Part model, mm, in its own coordinate system. Face numbers are marked on the shaded views. A direction names the side the tool comes from. Coordinates: 2 decimals unless noted, no trailing zeros. Loops run counter-clockwise (first coordinate to the right, second up) from the corner with the lowest first, then second, coordinate; pieces in that order, holes last. Notation, with made-up numbers: (-19, 71) -> (31, 71) arc R36 ccw to (31, 105) -> close; hole circle Ø8 at (61, 4). An arc over 180 degrees is marked (long way). One line per question, with ' | ' between items. Start each with the question number.
1) 3-axis set-ups, long thin cutter, end or side, ignore diameter. For the marked faces 1, 2, 3, 4 and 5: which of +Z, -Z, +X, -X, +Y, -Y reach the whole face in a straight line?
2) Cut at B-B (y = -2). List the corners of the cut face in (x, z), plus the area to 3 significant figures.
3) Probe L1, parallel to Z at x = -12.5, y = -29.8; L2, parallel to Y at x = 8, z = 50.95; L3, parallel to X at y = -30, z = 16. List the from-to ranges inside material, lowest first. Write a range as from..to.
4) Cut at D-D (x = 0). List the corners of the cut face in (y, z).
5) Drop flat-ended pins along their axis: pin 1 (6 mm diameter, centred on x = -10.5, z = 5, fed in from +Y); pin 2 (8 mm diameter, centred on x = -13.5, y = -12.5, fed in from +Z); pin 3 (5.5 mm diameter, centred on y = 1, z = 52.5, fed in from +X); pin 4 (2.5 mm diameter, centred on x = -8, y = 8, fed in from +Z). Give the stop position or say it passes through.
6) Two-plate mould, pull along Z, no slides. Class the marked faces 6, 7 and 8: released by +Z, released by -Z, zero draft, split by the parting line, or undercut.
7) Cut at A-A (x = 8). List the corners of the cut face in (y, z).
8) Cut at C-C (z = 0). List the corners of the cut face in (x, y), plus the area to 3 significant figures.
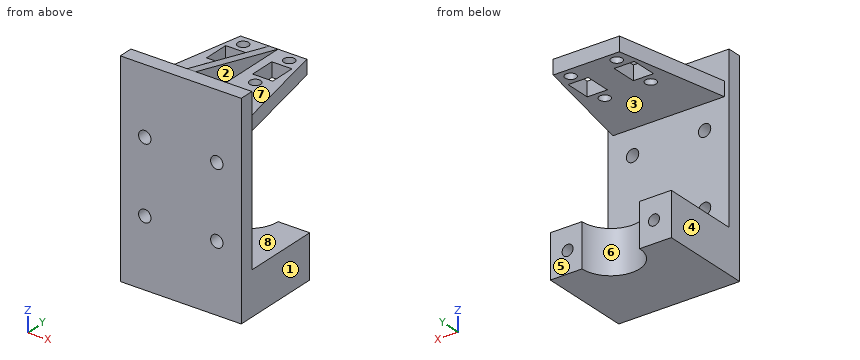
from build123d import *

# Parameters (mm, degrees)
MOTOR_MOUNT_SOLID_DEPTH              = 7.5
ENCODER_DISTANCE_SKETCH_W            = 50
ENCODER_DISTANCE_SKETCH_H            = 57
ENCODER_DISTANCE_SOLID_DEPTH         = 5
ENCODER_MOUNT_SKETCH_R               = 1.9
ENCODER_MOUNT_SKETCH_W               = 7
ENCODER_MOUNT_SKETCH_H               = 9
ENCODER_MOUNT_SOLID_DEPTH            = 5
MOTOR_CLAMP_MOUNTING_HOLES_SKETCH_R  = 1.9
MOTOR_CLAMP_MOUNTING_HOLES_CUT_DEPTH = 16
GUSSET_PLATE_SKETCH_W                = 50
GUSSET_PLATE_SKETCH_H                = 5
GUSSET_PLATE_SOLID_DEPTH             = 16.5
GUSSET_SOLID_DEPTH                   = 1.5
MOUNTING_PLATE_SKETCH_W              = 50
MOUNTING_PLATE_SKETCH_H              = 92
MOUNTING_PLATE_SKETCH_R              = 2.65
MOUNTING_PLATE_SOLID_DEPTH           = 5
MOUNTING_HOLES_CUT_DEPTH             = 101.440280764
MOUNTING_HOLES_CUT_DEPTH_BACK        = 101.440280764
MOUNTING_HOLE_SKETCH_R               = 2.65
MOUNTING_PLATE_TRIM_SKETCH_W         = 50
MOUNTING_PLATE_TRIM_SKETCH_H         = 13.5
MOUNTING_PLATE_TRIM_SKETCH_H_2       = 42
MOUNTING_PLATE_TRIM_SKETCH_W_2       = 23.5
MOUNTING_PLATE_TRIM_SKETCH_H_3       = 16.5
MOUNTING_PLATE_TRIM_CUT_DEPTH        = 2
CUT_EXTRUDE1_DEPTH                   = 102.917859083
CUT_EXTRUDE1_DEPTH_BACK              = 102.917859083
SKETCH2_W                            = 50
SKETCH2_H                            = 120
SKETCH2_W_2                          = 42
SKETCH2_H_2                          = 54.272597004
SKETCH3_W                            = 42
SKETCH3_H                            = 71.586450004
BOSS_EXTRUDE1_DEPTH                  = 5
CUT_EXTRUDE2_DEPTH                   = 78.722819275
CUT_EXTRUDE2_DEPTH_BACK              = 78.722819275
SKETCH4_R                            = 2.15


with BuildPart() as part:
    # Mouting Mount Sketch → Motor Mount Solid (new, symmetric)
    with BuildSketch(Plane.XY):
        with BuildLine():
            Line((-25, -55), (25, -55))
            Line((25, -55), (25, 0))
            Line((25, 0), (10, 0))
            ThreePointArc((10, 0), (0, -10), (-10, 0))
            Line((-10, 0), (-25, 0))
            Line((-25, 0), (-25, -55))
        make_face()
    extrude(amount=MOTOR_MOUNT_SOLID_DEPTH, both=True)

    # Encoder Distance Sketch → Encoder Distance Solid (add)
    with BuildSketch(Plane.XZ.offset(55)):
        with Locations((0, 21)):
            Rectangle(ENCODER_DISTANCE_SKETCH_W, ENCODER_DISTANCE_SKETCH_H)
    extrude(amount=ENCODER_DISTANCE_SOLID_DEPTH)

    # Encoder Mount Sketch → Encoder Mount Solid (add)
    with BuildSketch(Plane.XY.offset(49.5)):
        Polygon((-25, -60), (-25, -55), (-11.5, 11.5), (11.5, 11.5), (25, -55), (25, -60), align=None)
        with Locations((-8, 8)):
            Circle(ENCODER_MOUNT_SKETCH_R, mode=Mode.SUBTRACT)
        with Locations((8, 8)):
            Circle(ENCODER_MOUNT_SKETCH_R, mode=Mode.SUBTRACT)
        with Locations((-8, -8)):
            Circle(ENCODER_MOUNT_SKETCH_R, mode=Mode.SUBTRACT)
        with Locations((8, -8)):
            Circle(ENCODER_MOUNT_SKETCH_R, mode=Mode.SUBTRACT)
        with Locations((-8, 0)):
            Rectangle(ENCODER_MOUNT_SKETCH_W, ENCODER_MOUNT_SKETCH_H, mode=Mode.SUBTRACT)
        with Locations((8, 0)):
            Rectangle(ENCODER_MOUNT_SKETCH_W, ENCODER_MOUNT_SKETCH_H, mode=Mode.SUBTRACT)
    extrude(amount=ENCODER_MOUNT_SOLID_DEPTH)

    # Motor Clamp Mounting Holes Sketch → Motor Clamp Mounting Holes Cut (cut)
    with BuildSketch(Plane(origin=(0, 0, 0), x_dir=(1, 0, 0), z_dir=(0, 1, 0))):
        with Locations(Location((-15, 0, 0), (0, 0, 180))):
            Circle(MOTOR_CLAMP_MOUNTING_HOLES_SKETCH_R)
        with Locations(Location((15, 0, 0), (0, 0, 180))):
            Circle(MOTOR_CLAMP_MOUNTING_HOLES_SKETCH_R)
    extrude(amount=-MOTOR_CLAMP_MOUNTING_HOLES_CUT_DEPTH, mode=Mode.SUBTRACT)

    # Gusset Plate Sketch → Gusset Plate Solid (add)
    with BuildSketch(Plane.XY.offset(54.5)):
        with Locations((0, -57.5)):
            Rectangle(GUSSET_PLATE_SKETCH_W, GUSSET_PLATE_SKETCH_H)
    extrude(amount=GUSSET_PLATE_SOLID_DEPTH)

    # Gusset Sketch → Gusset Solid (add, symmetric)
    with BuildSketch(Plane(origin=(0, 0, 0), x_dir=(0, 0, -1), z_dir=(1, 0, 0))):
        Polygon((-54.5, 11.5), (-71, -55), (-54.5, -55), align=None)
    extrude(amount=GUSSET_SOLID_DEPTH, both=True)

    # Mounting Plate Sketch → Mounting Plate Solid (add)
    with BuildSketch(Plane(origin=(0, -55, 0), x_dir=(1, 0, 0), z_dir=(0, 1, 0))):
        with Locations((0, -25)):
            Rectangle(MOUNTING_PLATE_SKETCH_W, MOUNTING_PLATE_SKETCH_H)
        with Locations((-19, -65)):
            Circle(MOUNTING_PLATE_SKETCH_R, mode=Mode.SUBTRACT)
        with Locations((19, -65)):
            Circle(MOUNTING_PLATE_SKETCH_R, mode=Mode.SUBTRACT)
        with Locations(Location((-19, 15, 0), (0, 0, 270))):
            Circle(MOUNTING_PLATE_SKETCH_R, mode=Mode.SUBTRACT)
        with Locations(Location((19, 15, 0), (0, 0, 270))):
            Circle(MOUNTING_PLATE_SKETCH_R, mode=Mode.SUBTRACT)
    extrude(amount=-MOUNTING_PLATE_SOLID_DEPTH)

    # Mounting Hole Sketch → Mounting Holes Cut (cut, two sides: drawn at the far end of the back side and taken through both)
    with BuildSketch(Plane(origin=(0, -55, 0), x_dir=(1, 0, 0), z_dir=(0, 1, 0)).offset(-MOUNTING_HOLES_CUT_DEPTH_BACK)):
        with Locations(Location((-19, 15, 0), (0, 0, 270))):
            Circle(MOUNTING_HOLE_SKETCH_R)
        with Locations(Location((19, 15, 0), (0, 0, 270))):
            Circle(MOUNTING_HOLE_SKETCH_R)
        with Locations(Location((19, -65, 0), (0, 0, 90))):
            Circle(MOUNTING_HOLE_SKETCH_R)
        with Locations(Location((-19, -65, 0), (0, 0, 90))):
            Circle(MOUNTING_HOLE_SKETCH_R)
    extrude(amount=MOUNTING_HOLES_CUT_DEPTH + MOUNTING_HOLES_CUT_DEPTH_BACK, mode=Mode.SUBTRACT)

    # Mounting Plate Trim Sketch → Mounting Plate Trim Cut (cut)
    with BuildSketch(Plane(origin=(0, -55, 0), x_dir=(1, 0, 0), z_dir=(0, 1, 0))):
        with Locations((0, 14.25)):
            Rectangle(MOUNTING_PLATE_TRIM_SKETCH_W, MOUNTING_PLATE_TRIM_SKETCH_H)
        with Locations((0, -28.5)):
            Rectangle(MOUNTING_PLATE_TRIM_SKETCH_W, MOUNTING_PLATE_TRIM_SKETCH_H_2)
        with Locations((13.25, -62.75)):
            Rectangle(MOUNTING_PLATE_TRIM_SKETCH_W_2, MOUNTING_PLATE_TRIM_SKETCH_H_3)
        with Locations((-13.25, -62.75)):
            Rectangle(MOUNTING_PLATE_TRIM_SKETCH_W_2, MOUNTING_PLATE_TRIM_SKETCH_H_3)
    extrude(amount=-MOUNTING_PLATE_TRIM_CUT_DEPTH, mode=Mode.SUBTRACT)

    # Sketch2 → Cut-Extrude1 (cut, two sides: drawn at the far end of the back side and taken through both)
    with BuildSketch(Plane(origin=(0, 0, -7.5), x_dir=(-1, 0, 0), z_dir=(0, 0, -1)).offset(-CUT_EXTRUDE1_DEPTH_BACK)):
        Rectangle(SKETCH2_W, SKETCH2_H)
        Rectangle(SKETCH2_W_2, SKETCH2_H_2, mode=Mode.SUBTRACT)
    extrude(amount=CUT_EXTRUDE1_DEPTH + CUT_EXTRUDE1_DEPTH_BACK, mode=Mode.SUBTRACT)


with BuildPart() as cut_extrude1_piece_1:
    # of the separate pieces the step leaves, piece 1, a body of its own (cut_extrude1_pieces)
    add(part.part.solids().sort_by_distance((21, 0, 7.5))[0])



with BuildPart() as cut_extrude1_piece_2:
    # of the separate pieces the step leaves, piece 2, a body of its own (cut_extrude1_pieces)
    add(part.part.solids().sort_by_distance((-1.5, -27.136298502, 54.5))[0])


with BuildPart() as cut_extrude1_piece_1_1:
    add(cut_extrude1_piece_1.part)

    add(cut_extrude1_piece_2.part)  # Boss-Extrude1 merges Cut-Extrude1 piece 2
    # Sketch3 → Boss-Extrude1 (add)
    with BuildSketch(Plane.XZ.offset(27.136298502)):
        with Locations((0, 28.293225002)):
            Rectangle(SKETCH3_W, SKETCH3_H)
    extrude(amount=BOSS_EXTRUDE1_DEPTH)

    # Sketch4 → Cut-Extrude2 (cut, two sides: drawn at the far end of the back side and taken through both)
    with BuildSketch(Plane(origin=(0, -27.136298502, 0), x_dir=(1, 0, 0), z_dir=(0, 1, 0)).offset(-CUT_EXTRUDE2_DEPTH_BACK)):
        with Locations(Location((-12.5, -16, 0), (0, 0, 270))):
            Circle(SKETCH4_R)
        with Locations(Location((12.5, -16, 0), (0, 0, 270))):
            Circle(SKETCH4_R)
        with Locations(Location((-12.5, -41, 0), (0, 0, 270))):
            Circle(SKETCH4_R)
        with Locations(Location((12.5, -41, 0), (0, 0, 270))):
            Circle(SKETCH4_R)
    extrude(amount=CUT_EXTRUDE2_DEPTH + CUT_EXTRUDE2_DEPTH_BACK, mode=Mode.SUBTRACT)


solid = cut_extrude1_piece_1_1.part
Reported:
1) face 1: +Z, -Z, +X, +Y, -Y | face 2: +Z, +X, +Y | face 3: +X, -X, +Y | face 4: +Z, -Z, -X, +Y, -Y | face 5: -Z, +X, -X, +Y
2) outline: (-21, -7.5) -> (-9.8, -7.5) -> (-9.8, 7.5) -> (-21, 7.5) -> close; (-14.24, 49.5) -> (-11.5, 49.5) -> (-11.5, 54.5) -> (-14.24, 54.5) -> close; (-4.5, 49.5) -> (4.5, 49.5) -> (4.5, 54.5) -> (1.5, 54.5) -> (1.5, 57.85) -> (-1.5, 57.85) -> (-1.5, 54.5) -> (-4.5, 54.5) -> close; (9.8, -7.5) -> (21, -7.5) -> (21, 7.5) -> (9.8, 7.5) -> close; (11.5, 49.5) -> (14.24, 49.5) -> (14.24, 54.5) -> (11.5, 54.5) -> close; hole circle Ø3.8 at (-15, 0); hole circle Ø3.8 at (15, 0) | area: 396 mm²
3) L1: z = -7.5..13.85, 18.15..38.85, 43.15..64.09 | L2: y = -32.14..-9.9, -6.1..-4.5, 4.5..6.1, 9.9..11.5 | L3: x = -21..-14.65, -10.35..10.35, 14.65..21
4) outline: (-32.14, -7.5) -> (-10, -7.5) -> (-10, 7.5) -> (-27.14, 7.5) -> (-27.14, 49.5) -> (11.5, 49.5) -> (11.5, 54.5) -> (-27.14, 64.09) -> (-32.14, 64.09) -> close
5) pin 1: stops at y = 0 | pin 2: stops at z = 54.5 | pin 3: stops at x = 14.19 | pin 4: passes through
6) face 6: zero draft | face 7: released by +Z | face 8: undercut
7) outline: (-32.14, -7.5) -> (-6, -7.5) -> (-6, 7.5) -> (-27.14, 7.5) -> (-27.14, 49.5) -> (-9.9, 49.5) -> (-9.9, 54.5) -> (-27.14, 54.5) -> (-27.14, 64.09) -> (-32.14, 64.09) -> close; (-6.1, 49.5) -> (-4.5, 49.5) -> (-4.5, 54.5) -> (-6.1, 54.5) -> close; (4.5, 49.5) -> (6.1, 49.5) -> (6.1, 54.5) -> (4.5, 54.5) -> close; (9.9, 49.5) -> (11.5, 49.5) -> (11.5, 54.5) -> (9.9, 54.5) -> close
8) outline: (-21, -32.14) -> (21, -32.14) -> (21, 0) -> (16.9, 0) -> (16.9, -16) -> (13.1, -16) -> (13.1, 0) -> (10, 0) arc R10 cw to (-10, 0) -> (-13.1, 0) -> (-13.1, -16) -> (-16.9, -16) -> (-16.9, 0) -> (-21, 0) -> close | area: 1,070 mm²
